```python
from build123d import *

# Parameters (mm, degrees)
SKETCH_1_W          = 77
SKETCH_1_H          = 33
EXTRUDE_1_DEPTH     = 77
CUT_EXTRUDE_1_DEPTH = 73
SKETCH_3_R          = 1.7
CUT_EXTRUDE_2_DEPTH = 93.196800378
CUT_EXTRUDE_3_REACH = 112.137
SKETCH_5_W          = 10
SKETCH_5_H          = 15.5
CUT_EXTRUDE_4_DEPTH = 85.163531427
SKETCH_6_W          = 15.75
SKETCH_6_H          = 28
CUT_EXTRUDE_5_DEPTH = 59.5
FILLET_1_R          = 1


with BuildPart() as part:
    # ｽｹｯﾁ1 → ﾎﾞｽ - 押し出し1 (new body)
    with BuildSketch(Plane(origin=(0, 0, 0), x_dir=(1, 0, 0), z_dir=(0, 1, 0))):
        Rectangle(SKETCH_1_W, SKETCH_1_H)
    extrude(amount=EXTRUDE_1_DEPTH)

    # ｽｹｯﾁ2 → ｶｯﾄ - 押し出し1 (cut)
    with BuildSketch(Plane.XZ):
        with BuildLine():
            Line((12.75, 13.75), (-12.75, 13.75))
            ThreePointArc((-12.75, 13.75), (-16.992640687, 11.992640687), (-18.75, 7.75))
            Line((-18.75, 7.75), (-18.75, -7.75))
            ThreePointArc((-18.75, -7.75), (-16.992640687, -11.992640687), (-12.75, -13.75))
            Line((-12.75, -13.75), (12.75, -13.75))
            ThreePointArc((12.75, -13.75), (16.992640687, -11.992640687), (18.75, -7.75))
            Line((18.75, -7.75), (18.75, 7.75))
            ThreePointArc((18.75, 7.75), (16.992640687, 11.992640687), (12.75, 13.75))
        make_face()
    extrude(amount=-CUT_EXTRUDE_1_DEPTH, mode=Mode.SUBTRACT)

    # ｽｹｯﾁ3 → ｶｯﾄ - 押し出し2 (cut, through all)
    with BuildSketch(Plane.XY.offset(16.5)):
        with Locations((34.75, 3.5)):
            Circle(SKETCH_3_R)
        with Locations((34.75, 67)):
            Circle(SKETCH_3_R)
        with Locations((-34.75, 67)):
            Circle(SKETCH_3_R)
        with Locations((-34.75, 3.5)):
            Circle(SKETCH_3_R)
    extrude(amount=-CUT_EXTRUDE_2_DEPTH, mode=Mode.SUBTRACT)

    # ｽｹｯﾁ4 → ｶｯﾄ - 押し出し3 (cut, up to next)
    with BuildSketch(Plane.ZY.offset(38.5), mode=Mode.PRIVATE) as cut_extrude_3_sk1:
        with BuildLine():
            Line((6.5, 40), (-6.5, 40))
            ThreePointArc((-6.5, 40), (-10.742640687, 38.242640687), (-12.5, 34))
            Line((-12.5, 34), (-12.5, 0))
            Line((-12.5, 0), (12.5, 0))
            Line((12.5, 0), (12.5, 34))
            ThreePointArc((12.5, 34), (10.742640687, 38.242640687), (6.5, 40))
        make_face()
    cut_extrude_3_tool1 = extrude(cut_extrude_3_sk1.sketch, amount=-CUT_EXTRUDE_3_REACH, mode=Mode.PRIVATE) & part.part
    add(cut_extrude_3_tool1.solids().sort_by_distance((-38.5, 19.707157, 0))[0], mode=Mode.SUBTRACT)

    # ｽｹｯﾁ5 → ｶｯﾄ - 押し出し4 (cut, through all)
    with BuildSketch(Plane.XZ.offset(-73)):
        with Locations((7.75, 0)):
            Rectangle(SKETCH_5_W, SKETCH_5_H)
    extrude(amount=-CUT_EXTRUDE_4_DEPTH, mode=Mode.SUBTRACT)

    # ｽｹｯﾁ6 → ｶｯﾄ - 押し出し5 (cut)
    with BuildSketch(Plane(origin=(0, 0, 0), x_dir=(-1, 0, 0), z_dir=(0, -1, 0))):
        with Locations((-28.625, -0.5)):
            Rectangle(SKETCH_6_W, SKETCH_6_H)
    extrude(amount=-CUT_EXTRUDE_5_DEPTH, mode=Mode.SUBTRACT)

    # ﾌｨﾚｯﾄ1
    fillet_1_edges = [part.edges().sort_by_distance(p)[0] for p in [
        (38.5, 77, 0),
        (0, 77, -16.5),
        (-38.5, 77, 0),
        (0, 77, 16.5),
    ]]
    fillet(fillet_1_edges, radius=FILLET_1_R)


solid = part.part
```
Can you work these out from the model? Positions are in its coordinate system, mm. A direction names the side the tool comes from. Round coordinates to 2 decimals unless told otherwise and drop trailing zeros. Loops run counter-clockwise (first coordinate to the right, second up) from the corner with the lowest first, then second, coordinate; pieces in that order, holes last. Notation, with made-up numbers: M 71.25,-18.5 L 98.25,-18.5 A16 cw 98.25,7.5 Z; hole C -15.5,53 d5. An arc over 180 degrees is marked long. Write item = value, one per line. Start each with the question number.
(1) Suppose I cut it at D-D on y = 45. Write out the boundary of the cut face in (x, z), plus the area to 3 significant figures.
(2) If we mould it in two halves opening along Z, with no side actions, what happens to faces 1 (the face through (0, 73, 0)), 2 (the face through (-1, 37, 16.5)), 3 (the face through (-36.1, 2.47, 14.53)), 4 (the face through (-27.612, 38.289, -10.696))? For each: released by +Z, released by -Z, zero draft, split by the parting line, or undercut.
(3) Which directions (+Z, -Z, +X, -X, +Y, -Y) give clear straight access to the entire face, cutting with the end or side of a thin tool? Please do faces 5 (the face through (20.75, 29, 1)), 6 (the face through (-28, 17, -12.5)), 7 (the face through (8, 75, 7.75)), 8 (the face through (-1, 77, 0)), 9 (the face through (-36.1, 2.47, -14.47)).
(4) I need wall thicknesses on line 1 along X through (y, z) = (67, 4); line 2 along Z through (x, y) = (-29.5, 15.5); line 3 along X through (y, z) = (24.5, -7). Which ranges of each line are inside material? Lowest first, please.
(5) Suppose I cut it at A-A on z = -4.5. Write out the boundary of the cut face in (x, y), plus the area to 3 significant figures.
(6) Suppose I cut it at B-B on y = 67. Write out the boundary of the cut face in (x, z), plus the area to 3 significant figures.
(7) Suppose I cut it at C-C on x = -34.75. Write out the boundary of the cut face in (y, z), plus the area to 3 significant figures.
(8) I'm going to push flat-ended pins straight in: P1, Ø4, axis at x = -30.5, z = 2.5, coming from the -Y side; P2, Ø3, axis at x = -15.5, z = -8, coming from the -Y side; P3, Ø1, axis at y = 20.5, z = -3, coming from the -X side. Where does each tip first touch, or does it pass through?
Answer block:
q1.outline = M -38.5,-16.5 L 38.5,-16.5 L 38.5,16.5 L -38.5,16.5 Z; hole M -18.75,-7.75 A6 ccw -12.75,-13.75 L 12.75,-13.75 A6 ccw 18.75,-7.75 L 18.75,7.75 A6 ccw 12.75,13.75 L -12.75,13.75 A6 ccw -18.75,7.75 Z; hole M 20.75,-13.5 L 36.5,-13.5 L 36.5,14.5 L 20.75,14.5 Z
q1.area = 1,100 mm²
q2.face_1 = undercut
q2.face_2 = released by +Z
q2.face_3 = zero draft
q2.face_4 = undercut
q3.face_5 = -Y
q3.face_6 = -X, -Y
q3.face_7 = +Y, -Y
q3.face_8 = +Z, -Z, +X, -X, +Y
q3.face_9 = +Z, -Z
q4.line_1 = -38.5 to -36.45, -33.05 to -18.75, 18.75 to 33.05, 36.45 to 38.5
q4.line_2 = -16.5 to -12.5, 12.5 to 16.5
q4.line_3 = 18.75 to 20.75, 36.5 to 38.5
q5.outline = M -38.5,40 L -18.75,40 L -18.75,73 L 2.75,73 L 2.75,77 L -37.5,77 A1 ccw -38.5,76 Z; M 12.75,73 L 18.75,73 L 18.75,0 L 20.75,0 L 20.75,59.5 L 36.5,59.5 L 36.5,0 L 38.5,0 L 38.5,76 A1 ccw 37.5,77 L 12.75,77 Z; hole C -34.75,67 d3.4; hole C 34.75,67 d3.4
q5.area = 1,410 mm²
q6.outline = M -38.5,-16.5 L -36.45,-16.5 L -36.45,16.5 L -38.5,16.5 Z; M -33.05,-16.5 L 33.05,-16.5 L 33.05,16.5 L -33.05,16.5 Z; M 36.45,-16.5 L 38.5,-16.5 L 38.5,16.5 L 36.45,16.5 Z; hole M -18.75,-7.75 A6 ccw -12.75,-13.75 L 12.75,-13.75 A6 ccw 18.75,-7.75 L 18.75,7.75 A6 ccw 12.75,13.75 L -12.75,13.75 A6 ccw -18.75,7.75 Z
q6.area = 1,320 mm²
q7.outline = M 0,-16.5 L 1.8,-16.5 L 1.8,-12.5 L 0,-12.5 Z; M 0,12.5 L 1.8,12.5 L 1.8,16.5 L 0,16.5 Z; M 5.2,-16.5 L 65.3,-16.5 L 65.3,16.5 L 5.2,16.5 L 5.2,12.5 L 34,12.5 A6 cw 40,6.5 L 40,-6.5 A6 cw 34,-12.5 L 5.2,-12.5 Z; M 68.7,-16.5 L 76,-16.5 A1 ccw 77,-15.5 L 77,15.5 A1 ccw 76,16.5 L 68.7,16.5 Z
q7.area = 1,420 mm²
q8.P1 = 40
q8.P2 = 73
q8.P3 = 18.75
